Design review of the part built by this model. Coordinates are the model's own, in mm. Face numbers are marked on the shaded views. A direction names the side the tool comes from. Coordinates: 2 decimals unless noted, no trailing zeros. Loops run counter-clockwise (first coordinate to the right, second up) from the corner with the lowest first, then second, coordinate; pieces in that order, holes last. Notation, with made-up numbers: (-33, 17) -> (3, 17) arc R16 ccw to (3, 32) -> close; hole circle Ø5 at (66, 4.25). An arc over 180 degrees is marked (long way). Use a Markdown table: item, result. Add a question column.
Q1. Take a section at C-C on y = 0. Write out the cut boundary in (x, z).
Q2. Take a section at D-D on z = 1.5. Write out the cut boundary in (x, y).
Q3. For probe 1 along Y at (x, z) = (0, 4.5); probe 2 along X at (y, z) = (-7.6, 1.5); probe 3 along Y at (x, z) = (0, 2.55), list the stretches that pass through material, from the lowest coordinate up.
Q4. Clearance check with flat-ended pins moving along their axes: pin 1 Ø1.3 at (x, z) = (-3, 1.5) entering from -Y; pin 2 Ø1.7 at (x, y) = (-3.18, -2.46) entering from +Z; pin 3 Ø1 at (x, y) = (0, 6.22) entering from +Z; pin 4 Ø2.5 at (x, y) = (0, -4.53) entering from -Z. State where each tip first meets the part, or that it passes through.
Q5. Take a section at B-B on x = 0. Write out the cut boundary in (y, z), plus the area to 3 significant figures.
Q6. Draft analysis for pull direction Y (two halves, no side actions). For the marked faces 4, 5, 6 and 7, state which applies: pulls with the +Y half, pulls with the -Y half, needs draft (parallel to the pull), parting line crosses it, or undercut.
Q7. Take a section at A-A on y = 3.25. Write out the cut boundary in (x, z).
Q8. For the marked faces 1, 2 and 3, list the 3-axis set-ups (+Z, -Z, +X, -X, +Y, -Y) from which the entire face can be reached by the end or side of a thin tool; tool diameter is ignored.
from build123d import *

# Parameters (mm, degrees)
EXTRUDE_1_DEPTH     = 3
SKETCH_2_R          = 0.8
CUT_EXTRUDE_1_DEPTH = 3.5
SKETCH_6_R          = 3
SKETCH_6_R_2        = 1.05
CUT_EXTRUDE_2_DEPTH = 5
FILLET_1_R          = 0.5
CUT_EXTRUDE_4_DEPTH = 15.514169722
FILLET_2_R          = 0.5
SKETCH_13_R         = 1.25
SKETCH_13_R_2       = 0.8
EXTRUDE_2_DEPTH     = 6


with BuildPart() as part:
    # 草图1 → 凸台-拉伸1 (new body)
    with BuildSketch(Plane.XY):
        Polygon((-5, -9.782714055), (-5, -10.082714055), (5, -10.082714055), (5, -4.612414327), (5, 7.717285945), (-5, 7.717285945), align=None)
    extrude(amount=EXTRUDE_1_DEPTH)

    # 草图2 → 切除-拉伸1 (cut)
    with BuildSketch(Plane(origin=(0, -10.082714055, 0), x_dir=(-1, 0, 0), z_dir=(0, -1, 0))):
        with Locations(Location((3, -1.5, 0), (0, 0, 90))):
            Circle(SKETCH_2_R)
        with Locations(Location((-3, -1.5, 0), (0, 0, 270))):
            Circle(SKETCH_2_R)
    extrude(amount=-CUT_EXTRUDE_1_DEPTH, mode=Mode.SUBTRACT)

    # 草图6 → 切除-拉伸2 (cut)
    with BuildSketch(Plane(origin=(0, 0, 0), x_dir=(-1, 0, 0), z_dir=(0, 0, -1))):
        with Locations((0, 0.717285945)):
            Circle(SKETCH_6_R)
        with Locations((-3.181980515, 3.89926646)):
            Circle(SKETCH_6_R_2)
        with Locations((3.181980515, 3.89926646)):
            Circle(SKETCH_6_R_2)
        with Locations((3.181980515, -2.46469457)):
            Circle(SKETCH_6_R_2)
        with Locations((-3.181980515, -2.46469457)):
            Circle(SKETCH_6_R_2)
    extrude(amount=-CUT_EXTRUDE_2_DEPTH, mode=Mode.SUBTRACT)

    # 圆角1
    fillet_1_edges = [part.edges().sort_by_distance(p)[0] for p in [
        (-5, 7.717285945, 1.5),
        (5, 7.717285945, 1.5),
    ]]
    fillet(fillet_1_edges, radius=FILLET_1_R)

    # 草图12 → 切除-拉伸4 (cut, through all)
    with BuildSketch(Plane(origin=(5, 0, 0), x_dir=(0, 0, -1), z_dir=(1, 0, 0))):
        Polygon((-1.2, 7.717285945), (-1.2, -4.243803332), (0, -6.322264301), (0, 7.717285945), align=None)
    extrude(amount=-CUT_EXTRUDE_4_DEPTH, mode=Mode.SUBTRACT)

    # 圆角2
    fillet_2_edges = [part.edges().sort_by_distance(p)[0] for p in [
        (0, -4.243803332, 1.2),
        (0, -6.322264301, 0),
    ]]
    fillet(fillet_2_edges, radius=FILLET_2_R)

    # 草图13 → 凸台-拉伸2 (add)
    # profile 1 of 2: a face of its own
    with BuildSketch(Plane.XY.offset(3)):
        with Locations((0, 6.217285945)):
            Circle(SKETCH_13_R)
        with Locations((0, 6.217285945)):
            Circle(SKETCH_13_R_2, mode=Mode.SUBTRACT)
    # profile 2 of 2: a face of its own
    with BuildSketch(Plane.XY.offset(3)):
        with Locations((0, -4.532714055)):
            Circle(SKETCH_13_R)
        with Locations((0, -4.532714055)):
            Circle(SKETCH_13_R_2, mode=Mode.SUBTRACT)
    extrude(amount=EXTRUDE_2_DEPTH)


solid = part.part
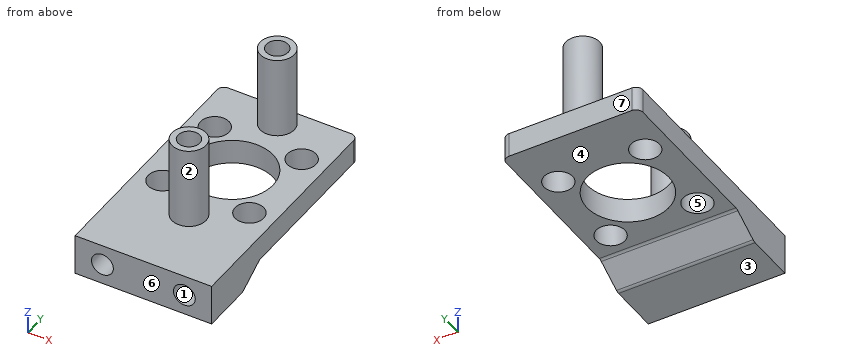
Answer list:
| question | item | result |
|---|---|---|
| 1 | outline | (-5, 1.2) -> (-2.91, 1.2) -> (-2.91, 3) -> (-5, 3) -> close; (2.91, 1.2) -> (5, 1.2) -> (5, 3) -> (2.91, 3) -> close |
| 2 | outline | (-5, -10.08) -> (-3.8, -10.08) -> (-3.8, -6.58) -> (-2.2, -6.58) -> (-2.2, -10.08) -> (2.2, -10.08) -> (2.2, -6.58) -> (3.8, -6.58) -> (3.8, -10.08) -> (5, -10.08) -> (5, 7.22) arc R0.5 ccw to (4.5, 7.72) -> (-4.5, 7.72) arc R0.5 ccw to (-5, 7.22) -> close; hole circle Ø2.1 at (-3.18, -2.46); hole circle Ø2.1 at (-3.18, 3.9); hole circle Ø6 at (0, 0.72); hole circle Ø2.1 at (3.18, -2.46); hole circle Ø2.1 at (3.18, 3.9) |
| 3 | probe 1 | -5.78 to -5.33, -3.73 to -3.28, 4.97 to 5.42, 7.02 to 7.47 |
| 3 | probe 2 | -5 to -3.8, -2.2 to 2.2, 3.8 to 5 |
| 3 | probe 3 | -10.08 to -2.28, 3.72 to 7.72 |
| 4 | pin 1 | y = -6.58 |
| 4 | pin 2 | through |
| 4 | pin 3 | z = 3 |
| 4 | pin 4 | z = 0.31 |
| 5 | outline | (-10.08, 0) -> (-6.46, 0) arc R0.5 ccw to (-6.21, 0.07) -> (-4.36, 1.13) arc R0.5 cw to (-4.11, 1.2) -> (-2.28, 1.2) -> (-2.28, 3) -> (-3.28, 3) -> (-3.28, 9) -> (-3.73, 9) -> (-3.73, 3) -> (-5.33, 3) -> (-5.33, 9) -> (-5.78, 9) -> (-5.78, 3) -> (-10.08, 3) -> close; (3.72, 1.2) -> (7.72, 1.2) -> (7.72, 3) -> (7.47, 3) -> (7.47, 9) -> (7.02, 9) -> (7.02, 3) -> (5.42, 3) -> (5.42, 9) -> (4.97, 9) -> (4.97, 3) -> (3.72, 3) -> close |
| 5 | area | 37.8 mm² |
| 6 | face 4 | needs draft |
| 6 | face 5 | undercut |
| 6 | face 6 | pulls with the -Y half |
| 6 | face 7 | pulls with the +Y half |
| 7 | outline | (-5, 1.2) -> (-4.01, 1.2) -> (-4.01, 3) -> (-5, 3) -> close; (-2.36, 1.2) -> (-1.61, 1.2) -> (-1.61, 3) -> (-2.36, 3) -> close; (1.61, 1.2) -> (2.36, 1.2) -> (2.36, 3) -> (1.61, 3) -> close; (4.01, 1.2) -> (5, 1.2) -> (5, 3) -> (4.01, 3) -> close |
| 8 | face 1 | -Y |
| 8 | face 2 | +Z |
| 8 | face 3 | -Z, +X, -X, +Y, -Y |
